Can you work these out from the model? Positions are in its coordinate system, mm. Give positions to 0.01 mm unless a question says otherwise; leave off trailing zeros. Order: outer loops, then holes, each group sorted by start corner. A loop starts at its lowest first (then second) coordinate and runs counter-clockwise, first axis right, second up. Notation, with made-up numbers: M -20.5,18 L -10.5,18 A15 cw -10.5,46 Z; hole C 49,-37.75 d1. An arc over 180 degrees is marked long. Use a Markdown table: item, result. Add a question column.
from build123d import *

# Parameters (mm, degrees)
CROQUIS1_R              = 11
CROQUIS1_R_2            = 1.5
SALIENTE_EXTRUIR1_DEPTH = 20


with BuildPart() as part:
    # Croquis1 → Saliente-Extruir1 (new body)
    with BuildSketch(Plane.XY):
        with BuildLine():
            Line((19.934911271, -13.245043478), (44.365127053, -13.245043478))
            ThreePointArc((44.365127053, -13.245043478), (47.900660959, -11.780577384), (49.365127053, -8.245043478))
            Line((49.365127053, -8.245043478), (49.365127053, 11.454956522))
            ThreePointArc((49.365127053, 11.454956522), (48.364801216, 15.022297578), (45.708403889, 17.604956522))
            Line((45.708403889, 17.604956522), (17.470852565, 17.589387044))
            ThreePointArc((17.470852565, 17.589387044), (14.633403866, 15.127424661), (13.842612072, 11.454956522))
            Line((13.842612072, 11.454956522), (13.842612072, -6.245043478))
            ThreePointArc((13.842612072, -6.245043478), (15.439014203, -11.006799955), (19.934911271, -13.245043478))
        make_face()
        with Locations(Location((27.865127053, 2.604956522, 0), (0, 0, 180))):
            Circle(CROQUIS1_R, mode=Mode.SUBTRACT)
        with Locations(Location((46.365127053, 2.454956522, 0), (0, 0, 180))):
            Circle(CROQUIS1_R_2, mode=Mode.SUBTRACT)
        with Locations(Location((46.365127053, 12.454956522, 0), (0, 0, 180))):
            Circle(CROQUIS1_R_2, mode=Mode.SUBTRACT)
        with Locations(Location((46.365127053, -7.545043478, 0), (0, 0, 180))):
            Circle(CROQUIS1_R_2, mode=Mode.SUBTRACT)
    extrude(amount=SALIENTE_EXTRUIR1_DEPTH)


solid = part.part
1. If we section it at D-D, the plane z = 10.5: List the corners of the cut face in (x, y) for me, then the cut area to 3 significant figures.
2. Will these pins go through, and if not, where does the flat tip stop? pin 1 (4 mm diameter, centred on x = 46.37, y = 12.45, fed in from +Z); pin 2 (3 mm diameter, centred on y = -10, z = 14.5, fed in from +X); pin 3 (5 mm diameter, centred on x = 22, z = 6.5, fed in from +Y); pin 4 (9 mm diameter, centred on y = 7, z = 7.5, fed in from -X).
3. If we section it at B-B, the plane x = 27: List the corners of the cut face in (y, z) for me.
4. I need wall thicknesses on L1, parallel to Y at x = 47.5, z = 2; L2, parallel to Y at x = 47, z = 15.75; L3, parallel to X at y = 1.5, z = 2.25. Which ranges of each line are inside material? Lowest first, please. Write a range as [from, to].
5. If we section it at A-A, the plane y = -5: List the corners of the cut face in (x, z) for me.
6. If we section it at C-C, the plane y = 13: List the corners of the cut face in (x, z) for me, then the cut area to 3 significant figures.
7. We'd pull the mould along Y, two halves only. Please class faces 1 (the face through (44.934, -7.996, 9.86)), 2 (the face through (47.86, -11.82, 9.86)): +Y half, -Y half, draft (parallel to the pull), parting line (faces both ways), or undercut.
Geometry results:
| question | item | result |
|---|---|---|
| 1 | outline | M 13.84,-6.25 A6.56 ccw 19.93,-13.25 L 44.37,-13.25 A5 ccw 49.37,-8.25 L 49.37,11.45 A7.12 ccw 45.71,17.6 L 17.47,17.59 A5.93 ccw 13.84,11.45 Z; hole C 27.87,2.6 d22; hole C 46.37,-7.55 d3; hole C 46.37,2.45 d3; hole C 46.37,12.45 d3 |
| 1 | area | 668 mm^2 |
| 2 | pin 1 | stops at z = 20 |
| 2 | pin 2 | stops at x = 49.36 |
| 2 | pin 3 | stops at y = 17.59 |
| 2 | pin 4 | stops at x = 13.84 |
| 3 | outline | M -13.25,0 L -8.36,0 L -8.36,20 L -13.25,20 Z; M 13.57,0 L 17.59,0 L 17.59,20 L 13.57,20 Z |
| 4 | L1 | y = [-12.14, -8.53], [-6.56, 1.47], [3.44, 11.47], [13.44, 16.19] |
| 4 | L2 | y = [-12.49, -8.9], [-6.19, 1.1], [3.81, 11.1], [13.81, 16.68] |
| 4 | L3 | x = [13.84, 16.92], [38.81, 45.21], [47.52, 49.37] |
| 5 | outline | M 13.84,0 L 19.92,0 L 19.92,20 L 13.84,20 Z; M 35.81,0 L 49.37,0 L 49.37,20 L 35.81,20 Z |
| 6 | outline | M 13.87,0 L 24.27,0 L 24.27,20 L 13.87,20 Z; M 31.46,0 L 44.97,0 L 44.97,20 L 31.46,20 Z; M 47.76,0 L 49.18,0 L 49.18,20 L 47.76,20 Z |
| 6 | area | 506 mm^2 |
| 7 | face 1 | undercut |
| 7 | face 2 | -Y half |
